```python
from build123d import *

# Parameters (mm, degrees)
BOSS_EXTRU_2_DEPTH      = 10
ESQUISSE2_W             = 4.4
ESQUISSE2_H             = 3.4
ENL_V_MAT_EXTRU_1_DEPTH = 6
ESQUISSE3_R             = 0.25
BOSS_EXTRU_3_DEPTH      = 2.5
ESQUISSE5_R             = 1.75
ENL_V_MAT_EXTRU_2_DEPTH = 1
ESQUISSE6_W             = 1.538533865
ESQUISSE6_H             = 0.4
ESQUISSE6_W_2           = 0.4
ESQUISSE6_H_2           = 1.538533865
ENL_V_MAT_EXTRU_3_DEPTH = 0.5


with BuildPart() as part:
    # Esquisse1 → Boss.-Extru.2 (new body)
    with BuildSketch(Plane.XY):
        Polygon((-7.7, 0), (0, 0), (0, 4.5), (-2, 8), (-6.5, 8), (-7.7, 4.5), align=None)
    extrude(amount=BOSS_EXTRU_2_DEPTH)

    # Esquisse2 → Enlèv. mat.-Extru.1 (cut)
    with BuildSketch(Plane.ZY.offset(7.7)):
        with Locations((2.6, 2.1)):
            Rectangle(ESQUISSE2_W, ESQUISSE2_H)
        with Locations((7.4, 2.1)):
            Rectangle(ESQUISSE2_W, ESQUISSE2_H)
    extrude(amount=-ENL_V_MAT_EXTRU_1_DEPTH, mode=Mode.SUBTRACT)

    # Esquisse3 → Boss.-Extru.3 (add)
    with BuildSketch(Plane(origin=(0, 0, 0), x_dir=(-1, 0, 0), z_dir=(0, -1, 0))):
        with Locations(Location((3.85, -2.5, 0), (0, 0, 90))):
            Circle(ESQUISSE3_R)
        with Locations(Location((3.85, -7.5, 0), (0, 0, 90))):
            Circle(ESQUISSE3_R)
    extrude(amount=BOSS_EXTRU_3_DEPTH)

    # Esquisse5 → Enlèv. mat.-Extru.2 (cut)
    with BuildSketch(Plane(origin=(0, 8, 0), x_dir=(1, 0, 0), z_dir=(0, 1, 0))):
        with Locations(Location((-4.25, -7.5, 0), (0, 0, 180))):
            Circle(ESQUISSE5_R)
        with Locations(Location((-4.25, -2.5, 0), (0, 0, 180))):
            Circle(ESQUISSE5_R)
    extrude(amount=-ENL_V_MAT_EXTRU_2_DEPTH, mode=Mode.SUBTRACT)

    # Esquisse6 → Enlèv. mat.-Extru.3 (cut)
    with BuildSketch(Plane(origin=(0, 7, 0), x_dir=(1, 0, 0), z_dir=(0, 1, 0))):
        with Locations((-5.219266933, -7.5)):
            Rectangle(ESQUISSE6_W, ESQUISSE6_H)
        with Locations((-4.25, -8.469266933)):
            Rectangle(ESQUISSE6_W_2, ESQUISSE6_H_2)
        with Locations((-3.280733067, -7.5)):
            Rectangle(ESQUISSE6_W, ESQUISSE6_H)
        with Locations((-4.25, -6.530733067)):
            Rectangle(ESQUISSE6_W_2, ESQUISSE6_H_2)
        with Locations((-4.25, -7.5)):
            Rectangle(ESQUISSE6_W_2, ESQUISSE6_H)
        with Locations((-4.25, -3.469266933)):
            Rectangle(ESQUISSE6_W_2, ESQUISSE6_H_2)
        with Locations((-4.25, -2.5)):
            Rectangle(ESQUISSE6_W_2, ESQUISSE6_H)
        with Locations((-3.280733067, -2.5)):
            Rectangle(ESQUISSE6_W, ESQUISSE6_H)
        with Locations((-4.25, -1.530733068)):
            Rectangle(ESQUISSE6_W_2, ESQUISSE6_H_2)
        with Locations((-5.219266933, -2.5)):
            Rectangle(ESQUISSE6_W, ESQUISSE6_H)
    extrude(amount=-ENL_V_MAT_EXTRU_3_DEPTH, mode=Mode.SUBTRACT)


solid = part.part
```
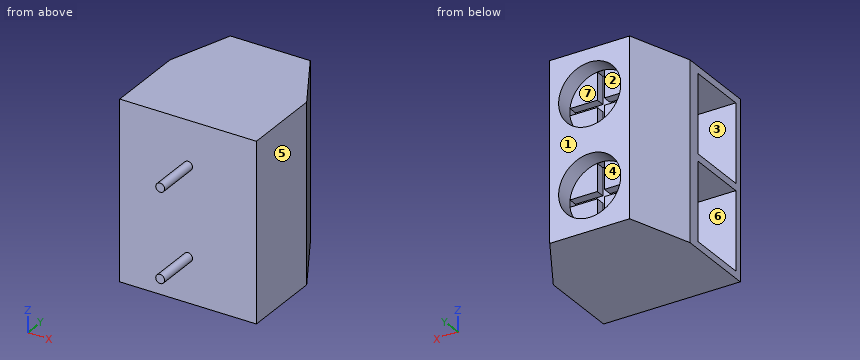
Verification items for the finished model (mm, model axes). Face numbers are marked on the shaded views. A direction names the side the tool comes from. Coordinates: 2 decimals unless noted, no trailing zeros. Loops run counter-clockwise (first coordinate to the right, second up) from the corner with the lowest first, then second, coordinate; pieces in that order, holes last. Notation, with made-up numbers: (19.5, 42.5) - (49.5, 42.5) arc R14 ccw to (49.5, 51.5) - close; hole circle Ø8 at (-33.75, -5). An arc over 180 degrees is marked (long way). Answer as a JSON object with one key per item and string values.
(1) Mould release check, pull along X, two halves, no side actions. Record for the marked faces 4, 5, 6 and 7: pulls with the +X half, pulls with the -X half, needs draft (parallel to the pull), parting line crosses it, or undercut.
Response:
{"face 4": "undercut", "face 5": "pulls with the +X half", "face 6": "needs draft", "face 7": "undercut"}
(2) Go/stop test with flat-tipped pins: pin 1 Ø0.6 at (y, z) = (7, 1.5) entering from +X; pin 2 Ø2.5 at (y, z) = (2.5, 3) entering from -X; pin 3 Ø1.5 at (x, y) = (-4, -1.5) entering from +Z. Record where each tip stops, or that it passes through.
Response:
{"pin 1": "stops at x = -1.26", "pin 2": "stops at x = -1.7", "pin 3": "stops at z = 7.75"}
(3) Cross-section at C-C, the plane y = 1.5. Record the boundary of the cut face in (x, z), then the cut area to 3 significant figures.
Response:
{"outline": "(-7.7, 0) - (0, 0) - (0, 10) - (-7.7, 10) - (-7.7, 9.6) - (-1.7, 9.6) - (-1.7, 5.2) - (-7.7, 5.2) - (-7.7, 4.8) - (-1.7, 4.8) - (-1.7, 0.4) - (-7.7, 0.4) - close", "area": "24.2 mm²"}
(4) Access from +Z, -Z, +X, -X, +Y, -Y to the whole of each face (thin tool, end or side, straight path). Record for the marked faces 1, 2 and 3.
Response:
{"face 1": "+Z, -Z, +X, -X, +Y", "face 2": "+Y", "face 3": "-X"}
(5) Cross-section at B-B, the plane z = 5. Record the boundary of the cut face in (x, y).
Response:
{"outline": "(-7.7, 0) - (0, 0) - (0, 4.5) - (-2, 8) - (-6.5, 8) - (-7.7, 4.5) - close"}
(6) Cross-section at D-D, the plane x = -5.25. Record the boundary of the cut face in (y, z).
Response:
{"outline": "(0, 0) - (8, 0) - (8, 1.06) - (7, 1.06) - (7, 2.3) - (6.5, 2.3) - (6.5, 2.7) - (7, 2.7) - (7, 3.94) - (8, 3.94) - (8, 6.06) - (7, 6.06) - (7, 7.3) - (6.5, 7.3) - (6.5, 7.7) - (7, 7.7) - (7, 8.94) - (8, 8.94) - (8, 10) - (0, 10) - close; hole (0.4, 0.4) - (3.8, 0.4) - (3.8, 4.8) - (0.4, 4.8) - close; hole (0.4, 5.2) - (3.8, 5.2) - (3.8, 9.6) - (0.4, 9.6) - close"}
(7) Cross-section at A-A, the plane x = -4.25. Count the separate pieces of the cut face and the enclosed holes in it, then the cut area to 3 significant figures.
Response:
{"separate pieces": "1", "enclosed holes": "2", "area": "39.6 mm²"}
(8) Scan lines: line 1 along Z through (x, y) = (-5.5, 2); line 2 along Z through (x, y) = (-4.25, 7.65); line 3 along Y through (x, z) = (-3.75, 4.75). Record each from-to range of solid material in increasing order.
Response:
{"line 1": "z = 0 to 0.4, 4.8 to 5.2, 9.6 to 10", "line 2": "z = 0 to 0.75, 4.25 to 5.75, 9.25 to 10", "line 3": "y = 0 to 0.4, 3.8 to 8"}
